from build123d import *

# Parameters (mm, degrees)
F1_DEPTH = 3.175
F2_R     = 1.7526
F3_DEPTH = 3.175
F4_R     = 1.7526
F5_DEPTH = 25.4
F6_W     = 5.842
F6_H     = 6.35
F7_DEPTH = 25.4


with BuildPart() as f1:
    # F0 (on Top) → F1 (new body)
    with BuildSketch(Plane.XY):
        Polygon((-5.2705, 3.175), (-11.1125, 3.175), (-11.1125, -3.175), (-5.2705, -3.175), (-5.2705, -4.7625), (5.2705, -4.7625), (5.2705, -3.175), (11.1125, -3.175), (11.1125, 3.175), (5.2705, 3.175), (5.2705, 4.7625), (-5.2705, 4.7625), align=None)
    extrude(amount=F1_DEPTH)

    # F2 (on face) → F3 (join, through all)
    with BuildSketch(Plane(origin=(0, 0, 0), x_dir=(1, 0, 0), z_dir=(0, 0, -1))):
        with BuildLine():
            Line((5.2705, 4.7625), (5.2705, 11.43))
            ThreePointArc((5.2705, 11.43), (0, 16.7005), (-5.2705, 11.43))
            Line((-5.2705, 11.43), (-5.2705, 4.7625))
            Line((-5.2705, 4.7625), (5.2705, 4.7625))
        make_face()
        with Locations((0, 11.43)):
            Circle(F2_R, mode=Mode.SUBTRACT)
    extrude(amount=-F3_DEPTH)

    # F4 (on face) → F5 (cut)
    with BuildSketch(Plane(origin=(0, 0, 0), x_dir=(1, 0, 0), z_dir=(0, 0, -1))):
        Circle(F4_R)
    extrude(amount=-F5_DEPTH, mode=Mode.SUBTRACT)

    # F6 (on face) → F7 (cut)
    with BuildSketch(Plane.XY.offset(3.175)):
        with Locations((-8.1915, 0)):
            Rectangle(F6_W, F6_H)
        with Locations((8.1915, 0)):
            Rectangle(F6_W, F6_H)
    extrude(amount=-F7_DEPTH, mode=Mode.SUBTRACT)


solid = f1.part
Verification items for the finished model (mm, model axes). Give positions to 0.01 mm unless a question says otherwise; leave off trailing zeros. Order: outer loops, then holes, each group sorted by start corner. A loop starts at its lowest first (then second) coordinate and runs counter-clockwise, first axis right, second up. Notation, with made-up numbers: M -10.75,44.25 L 15.25,44.25 A30 cw 15.25,73.25 Z; hole C 37.5,-3 d6. An arc over 180 degrees is marked long. Answer as a JSON object with one key per item and string values. Group by question number.
1) Cross-section at C-C (z = 1.4). Enter the section's corners in (x, y).
2) Cross-section at A-A (x = 0). Enter the section's corners in (y, z) (1 decimal), then the cut area to 3 significant figures.
3) Cross-section at D-D (y = 1.5). Enter the section's corners in (x, z) (1 decimal), then the cut area to 3 significant figures.
4) Mould release check, pull along X, two halves, no side actions. Record for faces 1 (the face through (1.67, -0.53, 1.57)), 2 (the face through (0, -6, 3.175)), 3 (the face through (-5.27, -3, 2)): released by +X, released by -X, zero draft, split by the parting line, or undercut.
5) Cross-section at B-B (y = -0.75). Enter the section's corners in (x, z) (1 decimal), then the cut area to 3 significant figures.
6) Scan lines: line 1 along Y through (x, z) = (0, 2); line 2 along X through (y, z) = (0, 2.2); line 3 along Y through (x, z) = (-1.5, 0.5). Record each from-to range of solid material in increasing order. Write a range as [from, to].
Result sheet:
{
 "1": {"outline": "M -5.27,-11.43 A5.27 ccw 5.27,-11.43 L 5.27,4.76 L -5.27,4.76 Z; hole C 0,-11.43 d3.51; hole C 0,0 d3.51"},
 "2": {"outline": "M -16.7,0 L -13.2,0 L -13.2,3.2 L -16.7,3.2 Z; M -9.7,0 L -1.8,0 L -1.8,3.2 L -9.7,3.2 Z; M 1.8,0 L 4.8,0 L 4.8,3.2 L 1.8,3.2 Z", "area": "45.9 mm2"},
 "3": {"outline": "M -5.3,0 L -0.9,0 L -0.9,3.2 L -5.3,3.2 Z; M 0.9,0 L 5.3,0 L 5.3,3.2 L 0.9,3.2 Z", "area": "27.7 mm2"},
 "4": {"face 1": "undercut", "face 2": "zero draft", "face 3": "released by -X"},
 "5": {"outline": "M -5.3,0 L -1.6,0 L -1.6,3.2 L -5.3,3.2 Z; M 1.6,0 L 5.3,0 L 5.3,3.2 L 1.6,3.2 Z", "area": "23.4 mm2"},
 "6": {"line 1": "y = [-16.7, -13.18], [-9.68, -1.75], [1.75, 4.76]", "line 2": "x = [-5.27, -1.75], [1.75, 5.27]", "line 3": "y = [-16.48, -12.34], [-10.52, -0.91], [0.91, 4.76]"}
}
